from build123d import *

# Parameters (mm, degrees)
F0_R          = 1
F1_DEPTH      = 3
F3_DEPTH      = 4
F3_DEPTH_BACK = 4
F4_R          = 5


with BuildPart() as f1:
    # F0 (on Top) → F1 (new body)
    with BuildSketch(Plane.XY):
        with BuildLine():
            ThreePointArc((-4.924908, -2.924908), (-4.339122, -4.339122), (-2.924908, -4.924908))
            Line((-2.924908, -4.924908), (2.924908, -4.924908))
            ThreePointArc((2.924908, -4.924908), (4.339122, -4.339122), (4.924908, -2.924908))
            Line((4.924908, -2.924908), (4.924908, 2.924908))
            ThreePointArc((4.924908, 2.924908), (4.339122, 4.339122), (2.924908, 4.924908))
            Line((2.924908, 4.924908), (-2.924908, 4.924908))
            ThreePointArc((-2.924908, 4.924908), (-4.339122, 4.339122), (-4.924908, 2.924908))
            Line((-4.924908, 2.924908), (-4.924908, -2.924908))
        make_face()
        with BuildLine():
            Line((-11.150462, -13.421226), (-2.924908, -4.924908))
            ThreePointArc((-2.924908, -4.924908), (-4.339122, -4.339122), (-4.924908, -2.924908))
            Line((-4.924908, -2.924908), (-13.421226, -11.150462))
            add(Edge.make_bspline(
                [(-16.544489, -13.448271), (-15.335972, -12.597233), (-14.270634, -12.001318), (-13.421226, -11.150462)],
                knots=[0, 0, 0, 0, 3.87746, 3.87746, 3.87746, 3.87746], degree=3))
            add(Edge.make_bspline(
                [(-16.544489, -13.448271), (-17.632553, -14.607294), (-18.696965, -16.286609), (-17.743413, -17.743413)],
                knots=[0, 0, 0, 0, 4.459169, 4.459169, 4.459169, 4.459169], degree=3))
            add(Edge.make_bspline(
                [(-13.448271, -16.544489), (-14.607294, -17.632553), (-16.286609, -18.696965), (-17.743413, -17.743413)],
                knots=[0, 0, 0, 0, 4.459169, 4.459169, 4.459169, 4.459169], degree=3))
            add(Edge.make_bspline(
                [(-13.448271, -16.544489), (-12.597233, -15.335972), (-12.001318, -14.270634), (-11.150462, -13.421226)],
                knots=[0, 0, 0, 0, 3.87746, 3.87746, 3.87746, 3.87746], degree=3))
        make_face()
        with BuildLine():
            ThreePointArc((4.924908, -2.924908), (4.339122, -4.339122), (2.924908, -4.924908))
            Line((2.924908, -4.924908), (11.150462, -13.421226))
            add(Edge.make_bspline(
                [(13.448271, -16.544489), (12.597233, -15.335972), (12.001318, -14.270634), (11.150462, -13.421226)],
                knots=[0, 0, 0, 0, 3.87746, 3.87746, 3.87746, 3.87746], degree=3))
            add(Edge.make_bspline(
                [(13.448271, -16.544489), (14.607294, -17.632553), (16.286609, -18.696965), (17.743413, -17.743413)],
                knots=[0, 0, 0, 0, 4.459169, 4.459169, 4.459169, 4.459169], degree=3))
            add(Edge.make_bspline(
                [(16.544489, -13.448271), (17.632553, -14.607294), (18.696965, -16.286609), (17.743413, -17.743413)],
                knots=[0, 0, 0, 0, 4.459169, 4.459169, 4.459169, 4.459169], degree=3))
            add(Edge.make_bspline(
                [(16.544489, -13.448271), (15.335972, -12.597233), (14.270634, -12.001318), (13.421226, -11.150462)],
                knots=[0, 0, 0, 0, 3.87746, 3.87746, 3.87746, 3.87746], degree=3))
            Line((13.421226, -11.150462), (4.924908, -2.924908))
        make_face()
        with BuildLine():
            Line((-13.421226, 11.150462), (-4.924908, 2.924908))
            ThreePointArc((-4.924908, 2.924908), (-4.339122, 4.339122), (-2.924908, 4.924908))
            Line((-2.924908, 4.924908), (-11.150462, 13.421226))
            add(Edge.make_bspline(
                [(-13.448271, 16.544489), (-12.597233, 15.335972), (-12.001318, 14.270634), (-11.150462, 13.421226)],
                knots=[0, 0, 0, 0, 3.87746, 3.87746, 3.87746, 3.87746], degree=3))
            add(Edge.make_bspline(
                [(-13.448271, 16.544489), (-14.607294, 17.632553), (-16.286609, 18.696965), (-17.743413, 17.743413)],
                knots=[0, 0, 0, 0, 4.459169, 4.459169, 4.459169, 4.459169], degree=3))
            add(Edge.make_bspline(
                [(-16.544489, 13.448271), (-17.632553, 14.607294), (-18.696965, 16.286609), (-17.743413, 17.743413)],
                knots=[0, 0, 0, 0, 4.459169, 4.459169, 4.459169, 4.459169], degree=3))
            add(Edge.make_bspline(
                [(-16.544489, 13.448271), (-15.335972, 12.597233), (-14.270634, 12.001318), (-13.421226, 11.150462)],
                knots=[0, 0, 0, 0, 3.87746, 3.87746, 3.87746, 3.87746], degree=3))
        make_face()
        with Locations((-15.324265, 15.324265)):
            Circle(F0_R, mode=Mode.SUBTRACT)
        with BuildLine():
            ThreePointArc((2.924908, 4.924908), (4.339122, 4.339122), (4.924908, 2.924908))
            Line((4.924908, 2.924908), (13.421226, 11.150462))
            add(Edge.make_bspline(
                [(16.544489, 13.448271), (15.335972, 12.597233), (14.270634, 12.001318), (13.421226, 11.150462)],
                knots=[0, 0, 0, 0, 3.87746, 3.87746, 3.87746, 3.87746], degree=3))
            add(Edge.make_bspline(
                [(16.544489, 13.448271), (17.632553, 14.607294), (18.696965, 16.286609), (17.743413, 17.743413)],
                knots=[0, 0, 0, 0, 4.459169, 4.459169, 4.459169, 4.459169], degree=3))
            add(Edge.make_bspline(
                [(13.448271, 16.544489), (14.607294, 17.632553), (16.286609, 18.696965), (17.743413, 17.743413)],
                knots=[0, 0, 0, 0, 4.459169, 4.459169, 4.459169, 4.459169], degree=3))
            add(Edge.make_bspline(
                [(13.448271, 16.544489), (12.597233, 15.335972), (12.001318, 14.270634), (11.150462, 13.421226)],
                knots=[0, 0, 0, 0, 3.87746, 3.87746, 3.87746, 3.87746], degree=3))
            Line((11.150462, 13.421226), (2.924908, 4.924908))
        make_face()
    extrude(amount=F1_DEPTH)

    # F2 (on Right) → F3 (join, two sides)
    with BuildSketch(Plane.YZ) as f3_sk:
        with BuildLine():
            Line((-6.486704, 6.056156), (-3.156722, 2.984606))
            Line((-3.156722, 2.984606), (3.611223, 2.984606))
            Line((3.611223, 2.984606), (3.611223, 6.190739))
            ThreePointArc((3.611223, 6.190739), (3.527195, 6.591982), (3.289231, 6.925793))
            Line((3.289231, 6.925793), (-1.19991, 11.066544))
            ThreePointArc((-1.19991, 11.066544), (-1.51395, 11.262901), (-1.877918, 11.331489))
            Line((-1.877918, 11.331489), (-4.193702, 11.331489))
            ThreePointArc((-4.193702, 11.331489), (-4.558258, 11.262671), (-4.872638, 11.065687))
            Line((-4.872638, 11.065687), (-6.487631, 9.572253))
            ThreePointArc((-6.487631, 9.572253), (-6.72492, 9.23872), (-6.808695, 8.838055))
            Line((-6.808695, 8.838055), (-6.808695, 6.79121))
            ThreePointArc((-6.808695, 6.79121), (-6.724667, 6.389967), (-6.486704, 6.056156))
        make_face()
    extrude(amount=F3_DEPTH)
    extrude(f3_sk.sketch, amount=-F3_DEPTH_BACK)

    # F4
    f4_edges = [f1.edges().sort_by_distance(p)[0] for p in [
        (4.924908, -2.924908, 1.5),
        (4.924908, 2.924908, 1.5),
        (2.924908, 4.924908, 1.5),
        (-2.924908, 4.924908, 1.5),
        (-4.924908, 2.924908, 1.5),
        (-4.924908, -2.924908, 1.5),
        (-2.924908, -4.924908, 1.5),
        (2.924908, -4.924908, 1.5),
    ]]
    fillet(f4_edges, radius=F4_R)


solid = f1.part
Can you work these out from the model? Positions are in its coordinate system, mm. A direction names the side the tool comes from. Give positions to 0.01 mm unless a question says otherwise; leave off trailing zeros. Loops run counter-clockwise (first coordinate to the right, second up) from the corner with the lowest first, then second, coordinate; pieces in that order, holes last. Notation, with made-up numbers: (53.5, -21) -> (57.5, -21) arc R11 cw to (57.5, -16) -> close; hole circle Ø4 at (46, 30.25). An arc over 180 degrees is marked (long way). Use one line per item in the form item = value.
1) If we section it at C-C (y = 1.5): Please give me the cut outline in (x, z).
Answers:
outline = (-4.97, 0) -> (4.97, 0) -> (4.97, 3) -> (4, 3) -> (4, 8.58) -> (-4, 8.58) -> (-4, 3) -> (-4.97, 3) -> close
2) Will these pins go through, and if not, where does the flat tip stop? pin 1 (3 mm diameter, centred on y = 10.5, z = 1.5, fed in from +X); pin 2 (1.2 mm diameter, centred on x = -15.32, y = 15.32, fed in from -Z); pin 3 (3.5 mm diameter, centred on x = -1.5, z = 4.5, fed in from +Y); pin 4 (1.3 mm diameter, centred on x = 0.5, z = 2, fed in from +Y).
Answers:
pin_1 = 14.43
pin_2 = through
pin_3 = 5.19
pin_4 = 4.94
3) I need wall thicknesses on line 1 along Z through (x, y) = (11, -10); line 2 along X through (y, z) = (0, 8.5); line 3 along X through (y, z) = (-10.5, 1). Which ranges of each line are inside material? Lowest first, please.
Answers:
line_1 = 0 to 3
line_2 = -4 to 4
line_3 = -12.75 to -8.32, 8.32 to 12.75
4) If we section it at B-B (y = 8.5): Please give me the cut outline in (x, z), plus the area to 3 significant figures.
Answers:
outline = (-10.68, 0) -> (-6.39, 0) -> (-6.39, 3) -> (-10.68, 3) -> close; (6.39, 0) -> (10.68, 0) -> (10.68, 3) -> (6.39, 3) -> close
area = 25.8 mm²
5) If we section it at A-A (x = 10.5): Please give me the cut outline in (y, z).
Answers:
outline = (-12.75, 0) -> (-8.32, 0) -> (-8.32, 3) -> (-12.75, 3) -> close; (8.32, 0) -> (12.75, 0) -> (12.75, 3) -> (8.32, 3) -> close
6) If we section it at D-D (z = 3.5): Please give me the cut outline in (x, y).
Answers:
outline = (-4, -3.72) -> (4, -3.72) -> (4, 3.61) -> (-4, 3.61) -> close
7) For faces 1 (the face through (-5.31, 2.73, 1.52)), 2 (the face through (0, 3.611, 5)), 3 (the face through (2.78, -5.33, 1.52)), 4 (the face through (7.82, 9.98, 1.48)), which set-ups out of +Z, -Z, +X, -X, +Y, -Y let a thin tool reach every point of the face, with its end or its side?
Answers:
face_1 = +Z, -Z, -X
face_2 = +Z, +X, -X, +Y
face_3 = -Z, -Y
face_4 = +Z, -Z, +Y
8) We'd pull the mould along Y, two halves only. Please class faces 5 (the face through (9.98, -7.82, 1.48)), 6 (the face through (0, 4.925, 1)), 7 (the face through (0.1, -5.7, 10.3)): released by +Y, released by -Y, zero draft, split by the parting line, or undercut.
Answers:
face_5 = undercut
face_6 = released by +Y
face_7 = released by -Y
